The drawing under review shows one solid part. Ordinate dimensions are in mm from its lowest x, y, z. A direction names the side the tool comes from. Coordinates: 2 decimals unless noted, no trailing zeros. Write each loop counter-clockwise with the first axis right and the second up, starting at its lowest first coordinate (ties: lowest second). Pieces come first, ordered by that corner, then holes. Notation, with made-up numbers: (87, -23.75) - (132, -23.75) arc R27 ccw to (132, 12.25) - close; hole circle Ø4 at (-13, -15.5). An arc over 180 degrees is marked (long way). Use a Markdown table: item, result.
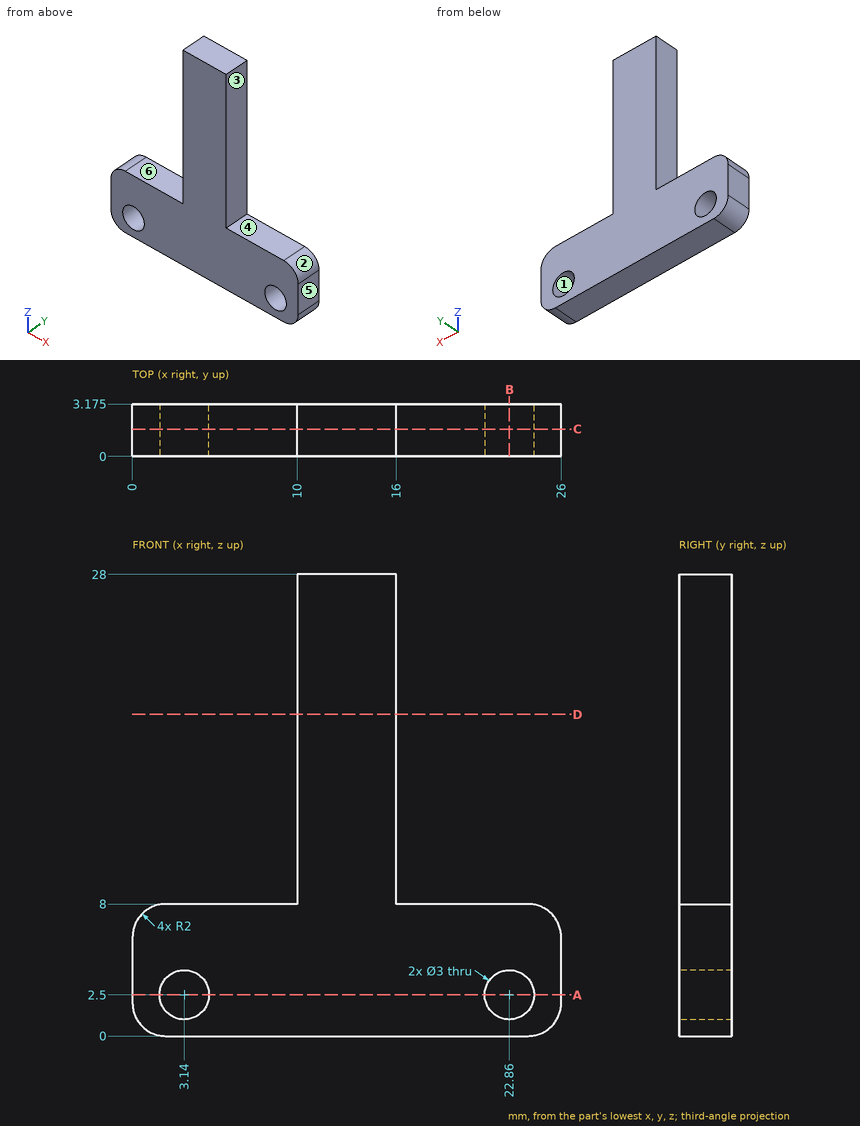
(1) For L1, parallel to X at y = 1.1, z = 2.5; L2, parallel to Z at x = 3.14, y = 2.5; L3, parallel to X at y = 2.4, z = 21.25, list the stretches that pass through material, from the lowest coordinate up. Write a range as from..to.
Determined:
| item | result |
|---|---|
| L1 | 0..1.64, 4.64..21.36, 24.36..26 |
| L2 | 0..1, 4..8 |
| L3 | 10..16 |
(2) For pin 1 (2.5 mm diameter, centred on x = 22.86, z = 2.5, fed in from +Y); pin 2 (1.6 mm diameter, centred on y = 1.5, z = 17.5, fed in from -X); pin 3 (10 mm diameter, centred on x = 19, z = 21, fed in from +Y) (3 decimals), all flat-tipped, find the tip position at first contact; note any pin that passes through.
Determined:
| item | result |
|---|---|
| pin 1 | through |
| pin 2 | x = 10 |
| pin 3 | y = 3.175 |
(3) Machinability: for the marked faces 4, 5 and 6, which of the approach directions +Z, -Z, +X, -X, +Y, -Y give a long, thin tool a straight path to every point of the face, cutting with its end or side? Answer none if there is none.
Determined:
| item | result |
|---|---|
| face 4 | +Z, +X, +Y, -Y |
| face 5 | +Z, -Z, +X, +Y, -Y |
| face 6 | +Z, -X, +Y, -Y |
(4) Take a section at D-D on z = 19.5. Write out the cut boundary in (x, y) (3 decimals), and give its area (4 significant figures).
Determined:
| item | result |
|---|---|
| outline | (10, 0) - (16, 0) - (16, 3.175) - (10, 3.175) - close |
| area | 19.05 mm2 |
(5) Take a section at C-C on y = 1.65. Write out the cut boundary in (x, z).
Determined:
| item | result |
|---|---|
| outline | (0, 2) arc R2 ccw to (2, 0) - (24, 0) arc R2 ccw to (26, 2) - (26, 6) arc R2 ccw to (24, 8) - (16, 8) - (16, 28) - (10, 28) - (10, 8) - (2, 8) arc R2 ccw to (0, 6) - close; hole circle Ø3 at (3.14, 2.5); hole circle Ø3 at (22.86, 2.5) |
(6) Take a section at A-A on z = 2.5. Write out the cut boundary in (x, y) (3 decimals), and give its area (3 significant figures).
Determined:
| item | result |
|---|---|
| outline | (0, 0) - (1.64, 0) - (1.64, 3.175) - (0, 3.175) - close; (4.64, 0) - (21.36, 0) - (21.36, 3.175) - (4.64, 3.175) - close; (24.36, 0) - (26, 0) - (26, 3.175) - (24.36, 3.175) - close |
| area | 63.5 mm2 |
(7) Take a section at B-B on x = 22.86. Write out the cut boundary in (y, z) (3 decimals).
Determined:
| item | result |
|---|---|
| outline | (0, 0) - (3.175, 0) - (3.175, 1) - (0, 1) - close; (0, 4) - (3.175, 4) - (3.175, 8) - (0, 8) - close |
(8) Draft analysis for pull direction Z (two halves, no side actions). For the marked faces 1, 2 and 3, state which applies: +Z half, -Z half, draft (parallel to the pull), parting line (faces both ways), or undercut.
Determined:
| item | result |
|---|---|
| face 1 | undercut |
| face 2 | +Z half |
| face 3 | draft |
